Source: CAD feature listing. Evaluate the final solid. Frame: model axes, mm. A direction names the side the tool comes from. Give positions to 0.01 mm unless a question says otherwise; leave off trailing zeros. Loops run counter-clockwise (first coordinate to the right, second up) from the corner with the lowest first, then second, coordinate; pieces in that order, holes last.
from build123d import *

# Parameters (mm, degrees)
F0_W     = 60
F0_H     = 25
F1_DEPTH = 30
F2_SIZE  = 5
F3_F1_R  = 5
F3_F2_R  = 5
F3_F3_R  = 5
F3_F4_R  = 5
F3_F5_R  = 5
F3_F6_R  = 5
F3_F7_R  = 5
F3_F8_R  = 5
F5_DEPTH = 25


with BuildPart() as f1:
    # F0 (on Top) → F1 (new body)
    with BuildSketch(Plane.XY):
        Rectangle(F0_W, F0_H)
    extrude(amount=F1_DEPTH)

    # F2
    f2_edges = [f1.edges().sort_by_distance(p)[0] for p in [
        (-30, 0, 30),
        (0, -12.5, 30),
        (30, 0, 30),
        (0, 12.5, 30),
    ]]
    chamfer(f2_edges, length=F2_SIZE)

    # F3: fillet of radius 5 on 8 edges, made by hand

    # F3_f1
    f3_f1_edges = [f1.edges().sort_by_distance(p)[0] for p in [
        (-30, 12.5, 12.5),
    ]]
    fillet(f3_f1_edges, radius=F3_F1_R)

    # F3_f2
    f3_f2_edges = [f1.edges().sort_by_distance(p)[0] for p in [
        (-30, -12.5, 12.5),
    ]]
    fillet(f3_f2_edges, radius=F3_F2_R)

    # F3_f3
    f3_f3_edges = [f1.edges().sort_by_distance(p)[0] for p in [
        (30, 12.5, 12.5),
    ]]
    fillet(f3_f3_edges, radius=F3_F3_R)

    # F3_f4
    f3_f4_edges = [f1.edges().sort_by_distance(p)[0] for p in [
        (-26.767766953, 9.267766953, 28.232233047),
    ]]
    fillet(f3_f4_edges, radius=F3_F4_R)

    # F3_f5
    f3_f5_edges = [f1.edges().sort_by_distance(p)[0] for p in [
        (-26.767766953, -9.267766953, 28.232233047),
    ]]
    fillet(f3_f5_edges, radius=F3_F5_R)

    # F3_f6
    f3_f6_edges = [f1.edges().sort_by_distance(p)[0] for p in [
        (30, -12.5, 12.5),
    ]]
    fillet(f3_f6_edges, radius=F3_F6_R)

    # F3_f7
    f3_f7_edges = [f1.edges().sort_by_distance(p)[0] for p in [
        (26.767766953, 9.267766953, 28.232233047),
    ]]
    fillet(f3_f7_edges, radius=F3_F7_R)

    # F3_f8
    f3_f8_edges = [f1.edges().sort_by_distance(p)[0] for p in [
        (26.767766953, -9.267766953, 28.232233047),
    ]]
    fillet(f3_f8_edges, radius=F3_F8_R)

    # F4 (on face) → F5 (cut)
    with BuildSketch(Plane(origin=(0, 0, 0), x_dir=(1, 0, 0), z_dir=(0, 0, -1))):
        with BuildLine():
            ThreePointArc((-25, -2.5), (-23.5355339059, -6.0355339059), (-20, -7.5))
            Line((-20, -7.5), (20, -7.5))
            ThreePointArc((20, -7.5), (23.5355339059, -6.0355339059), (25, -2.5))
            Line((25, -2.5), (25, 2.5))
            ThreePointArc((25, 2.5), (23.5355339059, 6.0355339059), (20, 7.5))
            Line((20, 7.5), (-20, 7.5))
            ThreePointArc((-20, 7.5), (-23.5355339059, 6.0355339059), (-25, 2.5))
            Line((-25, 2.5), (-25, -2.5))
        make_face()
    extrude(amount=-F5_DEPTH, mode=Mode.SUBTRACT)


solid = f1.part
1) Reachability of faces 1 (the cylindrical face through (-23.57, 6, 12.32)), 2 (the flat face through (28, 0, 27)) from +Z, -Z, +X, -X, +Y, -Y: full face, straight path, thin tool, end or side. Return the list, or none.
Checks:
face 1: -Z
face 2: +Z, +X, +Y, -Y
2) Ray query, probe 1 along X at (y, z) = (1.25, 11); probe 2 along Y at (x, z) = (18.5, 21); probe 3 along X at (y, z) = (-7.75, 17). Return the intervals inside material, ascending.
Checks:
probe 1: x = -30 to -25, 25 to 30
probe 2: y = -12.5 to -7.5, 7.5 to 12.5
probe 3: x = -29.99 to 29.99
3) Cut plane C-C (y = 1.5). Return loops of the section in (x, z).
Checks:
outline: (-30, 0) - (-25, 0) - (-25, 25) - (25, 25) - (25, 0) - (30, 0) - (30, 25) - (25, 30) - (-25, 30) - (-30, 25) - close
4) Cut plane A-A (z = 6). Return loops of the section in (x, y).
Checks:
outline: (-30, -7.5) arc R5 ccw to (-25, -12.5) - (25, -12.5) arc R5 ccw to (30, -7.5) - (30, 7.5) arc R5 ccw to (25, 12.5) - (-25, 12.5) arc R5 ccw to (-30, 7.5) - close; hole (-25, -2.5) arc R5 ccw to (-20, -7.5) - (20, -7.5) arc R5 ccw to (25, -2.5) - (25, 2.5) arc R5 ccw to (20, 7.5) - (-20, 7.5) arc R5 ccw to (-25, 2.5) - close
5) Pull-direction query (X, two-part tool) for faces 3 (the cylindrical face through (23.57, -6, 12.32)), 4 (the flat face through (0, -12.5, 12)), 5 (the cylindrical face through (26.032, -8.48, 28.046)); classes: released by +X, released by -X, zero draft, split by the parting line, or undercut.
Checks:
face 3: undercut
face 4: zero draft
face 5: released by +X
6) Cut plane B-B (x = 19). Return loops of the section in (y, z), and give its area (3 significant figures).
Checks:
outline: (-12.5, 0) - (-7.5, 0) - (-7.5, 25) - (7.5, 25) - (7.5, 0) - (12.5, 0) - (12.5, 25) - (7.5, 30) - (-7.5, 30) - (-12.5, 25) - close
area: 350 mm2
7) Contact query for flat-ended pins moving along their axis: P1, Ø4, axis at x = 16.5, y = 2, coming from the -Z side; P2, Ø3, axis at x = -10.5, z = 27, coming from the -Y side. Output: stop coordinate, or through.
Checks:
P1: stops at z = 25
P2: stops at y = -12
